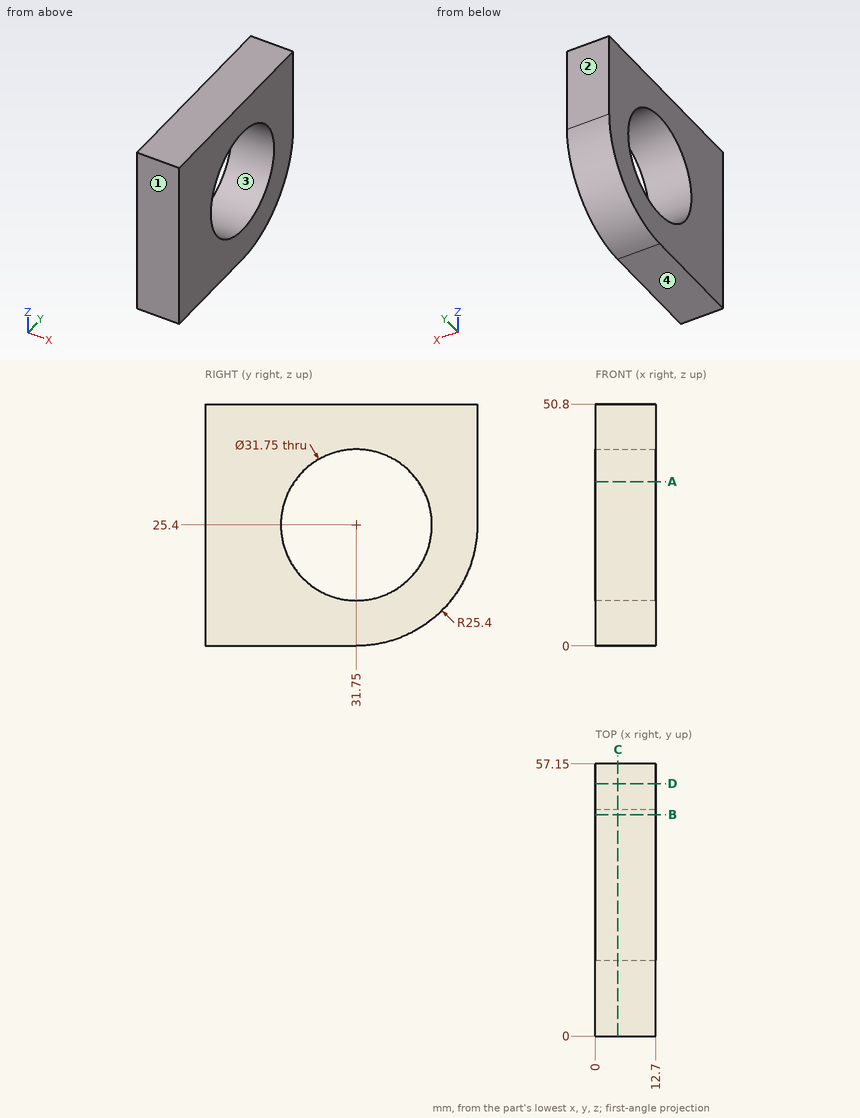
Source: three-view drawing plus pictorial views. Frame: mm from the lowest corner of the part. Coordinates: 2 decimals unless noted, no trailing zeros. Loops run counter-clockwise (first coordinate to the right, second up) from the corner with the lowest first, then second, coordinate; pieces in that order, holes last. Notation, with made-up numbers: (86, 23) - (121, 23) arc R22 cw to (121, 45) - close; hole circle Ø4 at (3.5, -37.5). An arc over 180 degrees is marked (long way). One line per question, with ' | ' between items.
1) Pull-direction query (Y, two-part tool) for the marked faces 1, 2, 3 and 4; classes: released by +Y, released by -Y, zero draft, split by the parting line, or undercut.
Report:
face 1: released by -Y | face 2: released by +Y | face 3: undercut | face 4: zero draft
2) Section C-C, the plane x = 4.75. Return loops of the section in (y, z) (3 decimals).
Report:
outline: (0, 0) - (31.75, 0) arc R25.4 ccw to (57.15, 25.4) - (57.15, 50.8) - (0, 50.8) - close; hole circle Ø31.75 at (31.75, 25.4)
3) Section D-D, the plane y = 53. Return loops of the section in (x, z).
Report:
outline: (0, 11.49) - (12.7, 11.49) - (12.7, 50.8) - (0, 50.8) - close
4) Section A-A, the plane z = 34.5. Return loops of the section in (x, y).
Report:
outline: (0, 0) - (12.7, 0) - (12.7, 18.74) - (0, 18.74) - close; (0, 44.76) - (12.7, 44.76) - (12.7, 57.15) - (0, 57.15) - close
5) Section B-B, the plane y = 46.5. Return loops of the section in (x, z).
Report:
outline: (0, 4.72) - (12.7, 4.72) - (12.7, 19.53) - (0, 19.53) - close; (0, 31.27) - (12.7, 31.27) - (12.7, 50.8) - (0, 50.8) - close
6) Line query: line 1 along Y through (x, z) = (7.5, 25.4) (3 decimals); line 2 along Z through (x, y) = (11.5, 32); line 3 along Z through (x, y) = (3.25, 21). Output: solid intervals per line, ascending.
Report:
line 1: y = 0 to 15.875, 47.625 to 57.15 | line 2: z = 0 to 9.53, 41.27 to 50.8 | line 3: z = 0 to 13.72, 37.08 to 50.8
